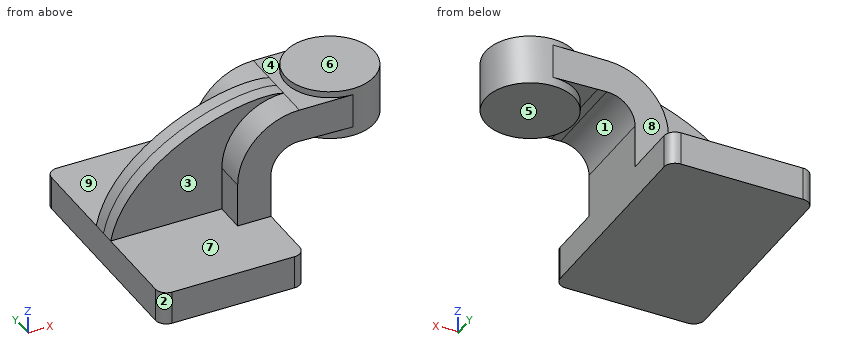
```python
from build123d import *

# Parameters (mm, degrees)
F1_DEPTH = 63.5
F2_DEPTH = 25.4
F3_DEPTH = 7.9375
F5_R     = 6.35


with BuildPart() as f1:
    # F0 (on Front) → F1 (new body, symmetric)
    with BuildSketch(Plane.XZ):
        Polygon((22.225, 9.525), (-41.275, 9.525), (-41.275, -9.525), (41.275, -9.525), (41.275, 9.525), align=None)
    extrude(amount=F1_DEPTH, both=True)

    # F0 (on Front) → F2 (join, symmetric)
    with BuildSketch(Plane.XZ):
        with BuildLine():
            Line((22.225, 34.4544437543), (22.225, 9.525))
            Line((22.225, 9.525), (41.275, 9.525))
            Line((41.275, 9.525), (41.275, 34.4544437543))
            ThreePointArc((41.275, 34.4544437543), (46.045587398, 45.7993829681), (57.4901364744, 50.3257994676))
            Line((57.4901364744, 50.3257994676), (57.4901364744, 69.3777874112))
            ThreePointArc((57.4901364744, 69.3777874112), (32.5748463013, 59.2701131123), (22.225, 34.4544437543))
        make_face()
        Polygon((88.0403167844, 69.3777874112), (62.6403167844, 69.3777874112), (62.6403167844, 50.2154267808), (88.0403167844, 49.6710834616), align=None)
        Polygon((62.6403167844, 69.3777874112), (57.4901364744, 69.3777874112), (57.4901364744, 50.3257994676), (62.6403167844, 50.2154267808), align=None)
    extrude(amount=F2_DEPTH, both=True)

    # F0 (on Front) → F3 (join, symmetric)
    with BuildSketch(Plane.XZ):
        with BuildLine():
            add(Edge.make_bspline(
                [(-41.275, 9.525), (-31.7188613117, 55.5080212653), (34.4085570037, 75.710179948), (57.4901364744, 69.3777874112)],
                knots=[0, 0, 0, 0, 115.4855330494, 115.4855330494, 115.4855330494, 115.4855330494], degree=3))
            Line((-41.275, 9.525), (22.225, 9.525))
            Line((22.225, 9.525), (22.225, 34.4544437543))
            ThreePointArc((22.225, 34.4544437543), (32.5748463013, 59.2701131123), (57.4901364744, 69.3777874112))
        make_face()
    extrude(amount=F3_DEPTH, both=True)

    # F0 (on Front) → F4 (revolve)
    with BuildSketch(Plane.XZ):
        Polygon((88.0403167844, 73.025), (88.0403167844, 69.3777874112), (88.0403167844, 49.6710834616), (88.0403167844, 44.45), (113.4403167844, 44.45), (113.4403167844, 73.025), align=None)
    revolve(axis=Axis((88.0403167844, 0, 58.7375), (0, 0, -1)))

    # F5
    f5_edges = [f1.edges().sort_by_distance(p)[0] for p in [
        (41.275, -63.5, 0),
        (-41.275, -63.5, 0),
        (-41.275, 63.5, 0),
        (41.275, 63.5, 0),
    ]]
    fillet(f5_edges, radius=F5_R)


solid = f1.part
```
Could you check a few things on this model? Use its own coordinates, in mm. Face numbers are marked on the shaded views. A direction names the side the tool comes from. Round coordinates to 2 decimals unless told otherwise and drop trailing zeros. Loops run counter-clockwise (first coordinate to the right, second up) from the corner with the lowest first, then second, coordinate; pieces in that order, holes last. Notation, with made-up numbers: (34, 1) - (79, 1) arc R25 ccw to (79, 24) - close; hole circle Ø10 at (-15, -10.75). An arc over 180 degrees is marked (long way). Use CSV: the item, a comma, the result in double quotes.
Item 1: Will these pins go through, and if not, where does the flat tip stop? pin 1 (8.5 mm diameter, centred on y = -14.5, z = 27, fed in from -X) (3 decimals); pin 2 (3 mm diameter, centred on y = 0.5, z = 18, fed in from -X); pin 3 (19 mm diameter, centred on y = 16.5, z = 24, fed in from -X).
Here are the results:
pin 1,"stops at x = 22.225"
pin 2,"stops at x = -39.34"
pin 3,"stops at x = -38.02"
Item 2: If we section it at A-A on z = 0.5: List the corners of the cut face in (x, y) for me (3 decimals), then the cut area to 3 significant figures.
Here are the results:
outline,"(-41.275, -57.15) arc R6.35 ccw to (-34.925, -63.5) - (34.925, -63.5) arc R6.35 ccw to (41.275, -57.15) - (41.275, 57.15) arc R6.35 ccw to (34.925, 63.5) - (-34.925, 63.5) arc R6.35 ccw to (-41.275, 57.15) - close"
area,"10,400 mm²"
Item 3: If we mould it in two halves opening along X, with no side actions, what happens to the marked faces 1, 2, 3 and 4? For each: pulls with the +X half, pulls with the -X half, needs draft (parallel to the pull), parting line crosses it, or undercut.
Here are the results:
face 1,"undercut"
face 2,"pulls with the -X half"
face 3,"needs draft"
face 4,"undercut"
Item 4: If we section it at B-B on x = 83: List the corners of the cut face in (y, z) for me (3 decimals).
Here are the results:
outline,"(-25.4, 49.779) - (-24.895, 49.779) - (-24.895, 44.45) - (24.895, 44.45) - (24.895, 49.779) - (25.4, 49.779) - (25.4, 69.378) - (24.895, 69.378) - (24.895, 73.025) - (-24.895, 73.025) - (-24.895, 69.378) - (-25.4, 69.378) - close"
Item 5: I need wall thicknesses on L1, parallel to Y at x = 41, z = 60; L2, parallel to Z at x = 19, y = 23 (3 decimals); L3, parallel to X at y = 31.5, z = 5 (3 decimals). Which ranges of each line are inside material? Lowest first, please. Write a range as [from, to].
Here are the results:
L1,"y = [-25.4, 25.4]"
L2,"z = [-9.525, 9.525]"
L3,"x = [-41.275, 41.275]"
Item 6: For the marked faces 5, 6, 7, 8 and 9, which set-ups out of +Z, -Z, +X, -X, +Y, -Y let a thin tool reach every point of the face, with its end or its side?
Here are the results:
face 5,"-Z, +X, +Y, -Y"
face 6,"+Z, +X, -X, +Y, -Y"
face 7,"+Z, -X, -Y"
face 8,"+Z, +X, -X, +Y"
face 9,"+Z, -X, +Y"
Item 7: If we section it at C-C on y = -30: List the corners of the cut face in (x, z) for me (3 decimals), then the cut area to 3 significant figures.
Here are the results:
outline,"(-41.275, -9.525) - (41.275, -9.525) - (41.275, 9.525) - (-41.275, 9.525) - close"
area,"1,570 mm²"
